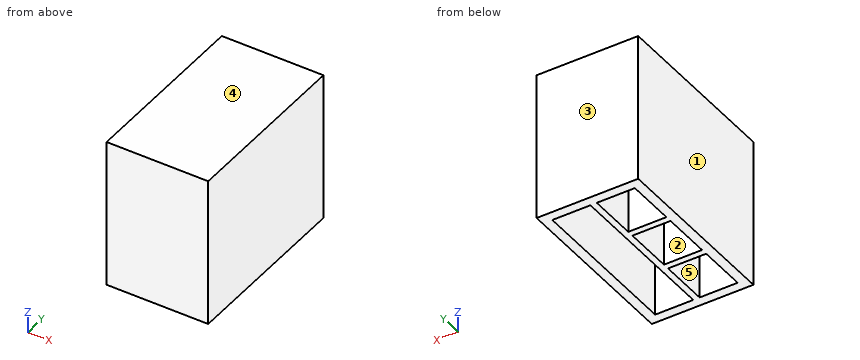
from build123d import *

# Parameters (mm, degrees)
F1_W     = 101.6
F1_H     = 177.8
F1_W_2   = 38.1
F1_H_2   = 48.6833333333
F1_H_3   = 158.75
F2_DEPTH = 139.7
F3_W     = 101.6
F3_H     = 177.8
F4_DEPTH = 9.525


# Not quite as in the source:
# - a variable given as a bare number and used for a length is read in inches; the dataset says mm whatever the document's units were


with BuildPart() as f2:
    # F1 (on Top) → F2 (new body)
    with BuildSketch(Plane.XY):
        with Locations((50.8, 88.9)):
            Rectangle(F1_W, F1_H)
        with Locations((28.575, 33.8666666667)):
            Rectangle(F1_W_2, F1_H_2, mode=Mode.SUBTRACT)
        with Locations((28.575, 88.9)):
            Rectangle(F1_W_2, F1_H_2, mode=Mode.SUBTRACT)
        with Locations((28.575, 143.9333333333)):
            Rectangle(F1_W_2, F1_H_2, mode=Mode.SUBTRACT)
        with Locations((73.025, 88.9)):
            Rectangle(F1_W_2, F1_H_3, mode=Mode.SUBTRACT)
    extrude(amount=F2_DEPTH)

    # F3 (on face) → F4 (join)
    with BuildSketch(Plane.XY.offset(139.7)):
        with Locations((50.8, 88.9)):
            Rectangle(F3_W, F3_H)
    extrude(amount=F4_DEPTH)


solid = f2.part
Source: CAD feature listing. Evaluate the final solid. Frame: model axes, mm. Face numbers are marked on the shaded views. A direction names the side the tool comes from. Coordinates: 2 decimals unless noted, no trailing zeros. Order: outer loops, then holes, each group sorted by start corner. A loop starts at its lowest first (then second) coordinate and runs counter-clockwise, first axis right, second up. Notation, with made-up numbers: M 88.25,-18 L 134.25,-18 A22 ccw 134.25,-1 Z; hole C 63.25,40.5 d11. An arc over 180 degrees is marked long. Write each question's results on one line, items separated by ' | '. Start each with the question number.
1. Draft query along Y for the marked faces 1, 2 and 3. Return one class per face: +Y half, -Y half, draft (parallel to the pull), parting line (faces both ways), or undercut.
2. Section B-B, the plane x = 15.5. Return the cut outline in (y, z) (3 decimals), then the cut area to 3 significant figures.
3. Section A-A, the plane z = 108.5. Return the cut outline in (x, y) (3 decimals), then the cut area to 3 significant figures.
4. Material intervals for L1, parallel to X at y = 104.5, z = 20.5 (3 decimals); L2, parallel to Y at x = 20, z = 29 (3 decimals); L3, parallel to Y at x = 85.5, z = 22.5 (3 decimals), sorted ascending.
5. Pin query (flat end, axial travel): pin 1 (19 mm diameter, centred on x = 69.5, y = 114, fed in from -Z). Return the tip coordinate at first contact, or that it passes through.
6. Reachability of the marked faces 4 and 5 from +Z, -Z, +X, -X, +Y, -Y: full face, straight path, thin tool, end or side. Return the list, or none.
7. Section C-C, the plane y = 127.5. Return the cut outline in (x, z) (3 decimals), then the cut area to 3 significant figures.
Solution:
1) face 1: draft | face 2: undercut | face 3: +Y half
2) outline: M 0,0 L 9.525,0 L 9.525,139.7 L 58.208,139.7 L 58.208,0 L 64.558,0 L 64.558,139.7 L 113.242,139.7 L 113.242,0 L 119.592,0 L 119.592,139.7 L 168.275,139.7 L 168.275,0 L 177.8,0 L 177.8,149.225 L 0,149.225 Z | area: 6,130 mm²
3) outline: M 0,0 L 101.6,0 L 101.6,177.8 L 0,177.8 Z; hole M 9.525,9.525 L 47.625,9.525 L 47.625,58.208 L 9.525,58.208 Z; hole M 9.525,64.558 L 47.625,64.558 L 47.625,113.242 L 9.525,113.242 Z; hole M 9.525,119.592 L 47.625,119.592 L 47.625,168.275 L 9.525,168.275 Z; hole M 53.975,9.525 L 92.075,9.525 L 92.075,168.275 L 53.975,168.275 Z | area: 6,450 mm²
4) L1: 0 to 9.525, 47.625 to 53.975, 92.075 to 101.6 | L2: 0 to 9.525, 58.208 to 64.558, 113.242 to 119.592, 168.275 to 177.8 | L3: 0 to 9.525, 168.275 to 177.8
5) pin 1: z = 139.7
6) face 4: +Z, +X, -X, +Y, -Y | face 5: -Z
7) outline: M 0,0 L 9.525,0 L 9.525,139.7 L 47.625,139.7 L 47.625,0 L 53.975,0 L 53.975,139.7 L 92.075,139.7 L 92.075,0 L 101.6,0 L 101.6,149.225 L 0,149.225 Z | area: 4,520 mm²
